Check sheet for the modelled part. Datum: model origin and axes. Units: mm. Face numbers are marked on the shaded views. A direction names the side the tool comes from. Coordinates: 2 decimals unless noted, no trailing zeros. Loops run counter-clockwise (first coordinate to the right, second up) from the corner with the lowest first, then second, coordinate; pieces in that order, holes last. Notation, with made-up numbers: (76.5, 48) - (87.5, 48) arc R29 ccw to (87.5, 69) - close; hole circle Ø1 at (46, 30.25). An arc over 180 degrees is marked (long way). Write each question's results on one line, items separated by ' | '. Start each with the question number.
1. Cross-section at A-A (y = 10). Record the cut outline in (x, z).
2. Tool access check on the marked faces 1, 2 and 3. Record the directions out of +Z, -Z, +X, -X, +Y, -Y that give a thin tool (end or side, any length) a straight path to the whole face; none if there is none.
3. Cross-section at D-D (y = 36.5). Record the cut outline in (x, z).
4. Gauge pin test, flat ends, axial feed: P1, Ø2, axis at x = 6.12, y = 66.49, coming from the +Z side (3 decimals); P2, Ø6, axis at x = 5, y = 131, coming from the -Z side; P3, Ø5, axis at x = 3, z = -3.5, coming from the +Y side. Record the tip position at first contact, or that the pin passes through.
5. Cross-section at C-C (z = -6.25). Record the cut outline in (x, y).
6. Cross-section at B-B (z = 1.25). Record the cut outline in (x, y), and give its area (3 significant figures).
7. Thickness scan on line 1 (X direction, y = 131, z = 1.95); line 2 (Y direction, x = 5.5, z = 0.25); line 3 (Y direction, x = 3.5, z = 4). Record the ranges inside material, lowest first. Write a range as [from, to].
```python
from build123d import *

# Parameters (mm, degrees)
SKETCH1_W           = 10
SKETCH1_H           = 141
SKETCH1_R           = 2.5
BOSS_EXTRUDE1_DEPTH = 5
SKETCH3_W           = 10
SKETCH3_H           = 35
BOSS_EXTRUDE3_DEPTH = 10
SKETCH4_R           = 1.2
CUT_EXTRUDE1_DEPTH  = 15
FILLET1_R           = 1


with BuildPart() as part:
    # Sketch1 → Boss-Extrude1 (new body)
    with BuildSketch(Plane.XY):
        with Locations((5, 70.5)):
            Rectangle(SKETCH1_W, SKETCH1_H)
        with Locations((5, 131)):
            Circle(SKETCH1_R, mode=Mode.SUBTRACT)
        with Locations((5, 10)):
            Circle(SKETCH1_R, mode=Mode.SUBTRACT)
    extrude(amount=BOSS_EXTRUDE1_DEPTH)

    # Sketch3 → Boss-Extrude3 (add)
    with BuildSketch(Plane(origin=(0, 0, 0), x_dir=(-1, 0, 0), z_dir=(0, 0, -1))):
        with Locations((-5, 72.121118493)):
            Rectangle(SKETCH3_W, SKETCH3_H)
    extrude(amount=BOSS_EXTRUDE3_DEPTH)

    # Sketch4 → Cut-Extrude1 (cut)
    with BuildSketch(Plane(origin=(0, 0, -10), x_dir=(-1, 0, 0), z_dir=(0, 0, -1))):
        with Locations((-6.118193933, 66.494048402)):
            Circle(SKETCH4_R)
        with Locations((-6.118193933, 76.394048402)):
            Circle(SKETCH4_R)
    extrude(amount=-CUT_EXTRUDE1_DEPTH, mode=Mode.SUBTRACT)

    # Fillet1
    fillet1_edges = [part.edges().sort_by_distance(p)[0] for p in [
        (0, 141, 2.5),
        (10, 141, 2.5),
        (10, 0, 2.5),
        (0, 0, 2.5),
    ]]
    fillet(fillet1_edges, radius=FILLET1_R)


solid = part.part
```
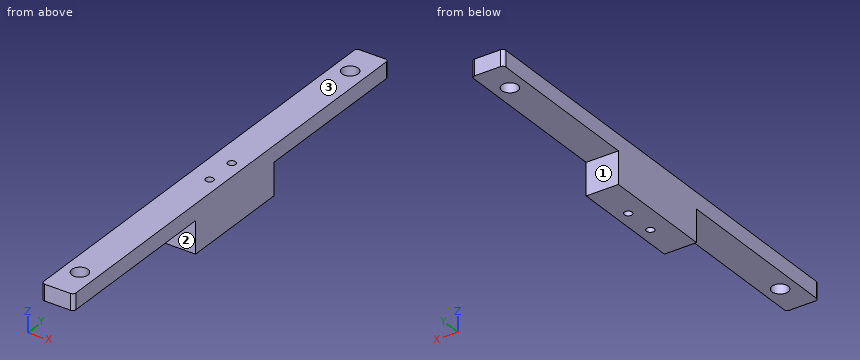
Established:
1) outline: (0, 0) - (2.5, 0) - (2.5, 5) - (0, 5) - close; (7.5, 0) - (10, 0) - (10, 5) - (7.5, 5) - close
2) face 1: -Z, +X, -X, +Y | face 2: -Z, +X, -X, -Y | face 3: +Z, +X, -X, +Y, -Y
3) outline: (0, 0) - (10, 0) - (10, 5) - (0, 5) - close
4) P1: through | P2: z = 0 | P3: y = 89.62
5) outline: (0, 54.62) - (10, 54.62) - (10, 89.62) - (0, 89.62) - close; hole circle Ø2.4 at (6.12, 66.49); hole circle Ø2.4 at (6.12, 76.39)
6) outline: (0, 1) arc R1 ccw to (1, 0) - (9, 0) arc R1 ccw to (10, 1) - (10, 140) arc R1 ccw to (9, 141) - (1, 141) arc R1 ccw to (0, 140) - close; hole circle Ø5 at (5, 10); hole circle Ø5 at (5, 131); hole circle Ø2.4 at (6.12, 66.49); hole circle Ø2.4 at (6.12, 76.39) | area: 1,360 mm^2
7) line 1: [0, 2.5], [7.5, 10] | line 2: [0, 7.55], [12.45, 65.47], [67.52, 75.37], [77.42, 128.55], [133.45, 141] | line 3: [0, 8], [12, 129], [133, 141]
